Source: CAD feature listing. Evaluate the final solid. Frame: model axes, mm. A direction names the side the tool comes from. Round coordinates to 2 decimals unless told otherwise and drop trailing zeros. Write each loop counter-clockwise with the first axis right and the second up, starting at its lowest first coordinate (ties: lowest second). Pieces come first, ordered by that corner, then holes. Notation, with made-up numbers: M -19.5,-4 L 7.5,-4 A23 ccw 7.5,24 Z; hole C 6.5,-2.5 d8. An arc over 180 degrees is marked long. Answer in a Markdown table with one row per item.
from build123d import *

# Parameters (mm, degrees)
SKETCH1_W                      = 6.866677178
SKETCH1_H                      = 28.893583938
BOSS_EXTRUDE1_DEPTH            = 11.43
SKETCH1_W_2                    = 6.571343666
SKETCH1_H_2                    = 36.38751909
BOSS_EXTRUDE1_2_DEPTH          = 11.43
BOSS_EXTRUDE2_DEPTH            = 20.574
CUT_EXTRUDE1_REACH             = 101.763
SKETCH2_R                      = 16.5
CUT_EXTRUDE1_DIRECTION_2_DEPTH = 35.052
CUT_EXTRUDE4_REACH             = 43.388
SKETCH3_R                      = 15.24
BOSS_EXTRUDE6_START            = -12.7
SKETCH15_R                     = 17.215000066
SKETCH15_R_2                   = 15.715000066
BOSS_EXTRUDE6_DEPTH            = 7.366
SKETCH16_R                     = 18.250000028
SKETCH16_R_2                   = 16.750000028
BOSS_EXTRUDE7_DEPTH            = 7


with BuildPart() as part:
    # Sketch1 → Boss-Extrude1 (new body, symmetric)
    with BuildSketch(Plane.XY):
        with Locations((-32.040465484, -10.249157812)):
            Rectangle(SKETCH1_W, SKETCH1_H)
    extrude(amount=BOSS_EXTRUDE1_DEPTH, both=True)



with BuildPart() as body_2:
    # Sketch1 → Boss-Extrude1 2 (new body, symmetric)
    with BuildSketch(Plane.XY):
        with Locations((-32.18813224, 51.873158257)):
            Rectangle(SKETCH1_W_2, SKETCH1_H_2)
    extrude(amount=BOSS_EXTRUDE1_2_DEPTH, both=True)


with BuildPart() as part_1:
    add(part.part)

    add(body_2.part)  # Boss-Extrude2 merges body 2
    # Sketch1_3 → Boss-Extrude2 (add, symmetric)
    with BuildSketch(Plane.XY):
        Polygon((-37.473804073, -26.695949781), (-35.473804073, -26.695949781), (-35.473804073, -24.695949781), (-35.473804073, 4.197634157), (-35.473804073, 33.679398712), (-35.473804073, 70.066917802), (-35.473804073, 75.066917802), (-37.473804073, 75.066917802), align=None)
    extrude(amount=BOSS_EXTRUDE2_DEPTH, both=True)

    # Sketch2 → Cut-Extrude1 (cut, up to next)
    with BuildSketch(Plane.XZ.offset(24.695949781), mode=Mode.PRIVATE) as cut_extrude1_sk1:
        with Locations((-15.773804073, 0)):
            Circle(SKETCH2_R)
    cut_extrude1_tool1 = extrude(cut_extrude1_sk1.sketch, amount=-CUT_EXTRUDE1_REACH, mode=Mode.PRIVATE) & part_1.part
    add(cut_extrude1_tool1.solids().sort_by_distance((-15.773804, -24.69595, 0))[0], mode=Mode.SUBTRACT)

    # Sketch2 → Cut-Extrude1 direction 2 (cut)
    with BuildSketch(Plane.XZ.offset(24.695949781)):
        with Locations((-15.773804073, 0)):
            Circle(SKETCH2_R)
    extrude(amount=CUT_EXTRUDE1_DIRECTION_2_DEPTH, mode=Mode.SUBTRACT)

    # Sketch3 → Cut-Extrude4 (cut, up to next)
    with BuildSketch(Plane.XZ.offset(-33.679398712), mode=Mode.PRIVATE) as cut_extrude4_sk1:
        with Locations((-15.883804073, 0)):
            Circle(SKETCH3_R)
    cut_extrude4_tool1 = extrude(cut_extrude4_sk1.sketch, amount=-CUT_EXTRUDE4_REACH, mode=Mode.PRIVATE) & part_1.part
    add(cut_extrude4_tool1.solids().sort_by_distance((-15.883804, 33.679399, 0))[0], mode=Mode.SUBTRACT)

    # Sketch15 → Boss-Extrude6 (add)
    with BuildSketch(Plane.XZ.offset(-33.679398712).offset(BOSS_EXTRUDE6_START)):
        with Locations((-15.883804073, 0)):
            Circle(SKETCH15_R)
        with Locations((-15.883804073, 0)):
            Circle(SKETCH15_R_2, mode=Mode.SUBTRACT)
    extrude(amount=-BOSS_EXTRUDE6_DEPTH)

    # Sketch16 → Boss-Extrude7 (add)
    with BuildSketch(Plane(origin=(0, 4.197634157, 0), x_dir=(1, 0, 0), z_dir=(0, 1, 0))):
        with Locations((-15.787690473, 0)):
            Circle(SKETCH16_R)
        with Locations((-15.787690473, 0)):
            Circle(SKETCH16_R_2, mode=Mode.SUBTRACT)
    extrude(amount=-BOSS_EXTRUDE7_DEPTH)


solid = part_1.part
Q1. Contact query for flat-ended pins moving along their axis: pin 1 Ø1.2 at (y, z) = (-14.5, 11) entering from +X; pin 2 Ø15 at (x, z) = (-19.5, 7) entering from -Y; pin 3 Ø1.5 at (x, z) = (-27.5, -14.5) entering from +Y; pin 4 Ø2 at (x, z) = (-31.5, 0.5) entering from +Y. Output: stop coordinate, or through.
Solutions:
| item | result |
|---|---|
| pin 1 | stops at x = -28.61 |
| pin 2 | passes through |
| pin 3 | stops at y = 4.2 |
| pin 4 | stops at y = 70.07 |
Q2. Material intervals for probe 1 along Y at (x, z) = (-33, -10); probe 2 along X at (y, z) = (6, 17); probe 3 along Z at (x, y) = (-32.5, 56.5), sorted ascending.
Solutions:
| item | result |
|---|---|
| probe 1 | y = -24.7 to 4.2, 33.68 to 70.07 |
| probe 2 | x = -37.47 to -35.47 |
| probe 3 | z = -11.43 to 11.43 |
Q3. Section A-A (z = 0). Return loops of the section in (x, y).
Solutions:
| item | result |
|---|---|
| outline | M -37.47,-26.7 L -35.47,-26.7 L -35.47,-24.7 L -32.27,-24.7 L -32.27,4.2 L -35.47,4.2 L -35.47,33.68 L -31.12,33.68 L -31.12,70.07 L -35.47,70.07 L -35.47,75.07 L -37.47,75.07 Z; M -0.17,46.38 L 1.33,46.38 L 1.33,53.75 L -0.17,53.75 Z; M 0.96,-2.8 L 2.46,-2.8 L 2.46,4.2 L 0.96,4.2 Z |
Q4. Access query for faces 1 (the cylindrical face through (-31.123, 51.618, 0.117)), 2 (the flat face through (-33, 33.679, 0)), 3 (the flat face through (-32, -10, 11.43)), 4 (the flat face through (-33, 70.067, 0)). Directions: +Z, -Z, +X, -X, +Y, -Y. A direction counts if a zero-diameter tool reaches every point of the face in a straight line with its end or side. Return the directions, or none.
Solutions:
| item | result |
|---|---|
| face 1 | +Y, -Y |
| face 2 | +Z, -Z, +X |
| face 3 | +Z, -Y |
| face 4 | +Z, -Z, +X, +Y |
Q5. Section B-B (y = -9). Return loops of the section in (x, z).
Solutions:
| item | result |
|---|---|
| outline | M -37.47,-20.57 L -35.47,-20.57 L -35.47,-11.43 L -28.61,-11.43 L -28.61,-10.37 A16.5 cw -28.61,10.37 L -28.61,11.43 L -35.47,11.43 L -35.47,20.57 L -37.47,20.57 Z |
Q6. Section D-D (z = -6.5). Return loops of the section in (x, y).
Solutions:
| item | result |
|---|---|
| outline | M -37.47,-26.7 L -35.47,-26.7 L -35.47,-24.7 L -30.94,-24.7 L -30.94,4.2 L -35.47,4.2 L -35.47,33.68 L -29.67,33.68 L -29.67,70.07 L -35.47,70.07 L -35.47,75.07 L -37.47,75.07 Z; M -1.58,46.38 L 0.06,46.38 L 0.06,53.75 L -1.58,53.75 Z; M -0.35,-2.8 L 1.27,-2.8 L 1.27,4.2 L -0.35,4.2 Z |
Q7. Pull-direction query (Y, two-part tool) for faces 5 (the flat face through (-28.902, 51.6, -8.5)), 6 (the flat face through (-32, 52, -11.43)), 7 (the flat face through (-36, 75.067, 0)); classes: pulls with the +Y half, pulls with the -Y half, needs draft (parallel to the pull), parting line crosses it, or undercut.
Solutions:
| item | result |
|---|---|
| face 5 | undercut |
| face 6 | needs draft |
| face 7 | pulls with the +Y half |
Q8. Section C-C (x = -21.5). Return loops of the section in (y, z).
Solutions:
| item | result |
|---|---|
| outline | M -2.8,-17.33 L 4.2,-17.33 L 4.2,-15.75 L -2.8,-15.75 Z; M -2.8,15.75 L 4.2,15.75 L 4.2,17.33 L -2.8,17.33 Z; M 46.38,-16.27 L 53.75,-16.27 L 53.75,-14.68 L 46.38,-14.68 Z; M 46.38,14.68 L 53.75,14.68 L 53.75,16.27 L 46.38,16.27 Z |
